Part model, mm, in its own coordinate system. A direction names the side the tool comes from. Give positions to 0.01 mm unless a question says otherwise; leave off trailing zeros. Order: outer loops, then holes, each group sorted by start corner. A loop starts at its lowest first (then second) coordinate and runs counter-clockwise, first axis right, second up. Notation, with made-up numbers: (46, 39) - (84, 39) arc R21 cw to (84, 76) - close; hole circle Ø10 at (-40, 80). An arc over 180 degrees is marked (long way). One line per item, written item: value.
```python
from build123d import *

# Parameters (mm, degrees)
SKETCH1_R      = 3.555
EXTRUDE1_DEPTH = 1.27
ICE1_DEPTH     = 6.35
SKETCH3_R      = 2.5
ICE2_DEPTH     = 8.62
SKETCH4_R      = 1
ICE3_DEPTH     = 0.2


with BuildPart() as part:
    # Sketch1 → Extrude1 (new body)
    with BuildSketch(Plane.XY):
        Circle(SKETCH1_R)
    extrude(amount=-EXTRUDE1_DEPTH)

    # Sketch2 → ICE1 (add)
    with BuildSketch(Plane.XY):
        Polygon((4.543746619, 0), (2.271873309, 3.935), (-2.271873309, 3.935), (-4.543746619, 0), (-2.271873309, -3.935), (2.271873309, -3.935), align=None)
    extrude(amount=ICE1_DEPTH)

    # Sketch3 → ICE2 (cut, through all)
    with BuildSketch(Plane.XY.offset(6.35)):
        with Locations((0, 0.79)):
            Circle(SKETCH3_R)
    extrude(amount=-ICE2_DEPTH, mode=Mode.SUBTRACT)

    # Sketch4 → ICE3 (cut)
    with BuildSketch(Plane(origin=(0, 3.935, 0), x_dir=(1, 0, 0), z_dir=(0, 1, 0))):
        with Locations((0, -3.175)):
            Circle(SKETCH4_R)
    extrude(amount=-ICE3_DEPTH, mode=Mode.SUBTRACT)

    # Sketch5 → RevCut1 (revolve, cut)
    with BuildSketch(Plane(origin=(0, 0, 0), x_dir=(-0.866025404, -0.5, 0), z_dir=(-0.5, 0.866025404, 0))):
        Polygon((-3.935, 6.35), (-10.285, 0), (-10.285, 6.35), align=None)
    revolve(axis=Axis((0, 0, 0), (0, 0, 1)), mode=Mode.SUBTRACT)


solid = part.part
```
1) Pin check, flat tip, straight feed: pin 1 (3 mm diameter, centred on y = 2.5, z = 5.5, fed in from -X). Stop position of the tip, or through.
Outcome:
pin 1: stops at x = -3.97
2) Cut at A-A, the plane z = 4.5. Give the cut face in (x, y) (3 decimals), then the cut area to 3 significant figures.
Outcome:
outline: (-4.544, 0) - (-2.272, -3.935) - (2.272, -3.935) - (4.544, 0) - (2.272, 3.935) - (-2.272, 3.935) - close; hole circle Ø5 at (0, 0.79)
area: 34.0 mm^2
3) Which spindle directions (+Z, -Z, +X, -X, +Y, -Y) get a long thin tool onto all of the face, cutting with end or side? Do faces 1 (the cylindrical face through (3.39, 1.07, -0.63)), 2 (the conical face through (2.05, 3.531, 6.202)). Say none if no direction does.
Outcome:
face 1: -Z
face 2: +Z, +X, +Y
4) Drill centre lines: line 1 along Y through (x, z) = (0, 4.75) (3 decimals); line 2 along Y through (x, z) = (0, 3) (3 decimals); line 3 along Z through (x, y) = (0, 3.8) (3 decimals). Where is each one in solid material? Low to high. Write a range as from..to.
Outcome:
line 1: y = -3.935..-1.71, 3.29..3.935
line 2: y = -3.935..-1.71, 3.29..3.735
line 3: z = 0..2.175, 4.175..6.35
5) Mould opens along X. For faces 3 (the conical face through (-2.05, -3.531, 6.202)), 4 (the flat face through (0, -2, -1.27)), 5 (the flat face through (0, 3.735, 3)) say: released by +X, released by -X, zero draft, split by the parting line, or undercut.
Outcome:
face 3: released by -X
face 4: zero draft
face 5: undercut
